Autodesk Inventor part; units mm, degrees
ref_plane "YZ Plane" through (0, 0, 0) normal (1, 0, 0) x (0, 1, 0)
ref_plane "XZ Plane" through (0, 0, 0) normal (0, 1, 0) x (-1, 0, 0)
ref_plane "XY Plane" through (0, 0, 0) normal (0, 0, 1) x (1, 0, 0)
sketch "Sketch1" plane through (0, 0, 0) normal (0, 0, 1) x (1, 0, 0)
  line L0 (0, 0) -> (95, 0)
  line L1 (95, 0) -> (95, 20)
  line L2 (95, 20) -> (0, 20)
  line L3 (0, 20) -> (0, 0)
  line L4 (8.5, 14.5) -> (14.5, 14.5)
  line L5 (18, 10.2244) -> (18, 9.7756)
  line L6 (14.5, 5.5) -> (8.5, 5.5)
  line L7 (5, 9.7756) -> (5, 10.2244)
  line L8 (11.5, 14.5) -> (8.5, 14.5)
  arc A0 (8.5, 14.5) -> (5, 10) centre (9.4986, 10.1122) ccw
  arc A1 (5, 10) -> (8.5, 5.5) centre (9.4986, 9.8878) ccw
  arc A2 (18, 10) -> (14.5, 14.5) centre (13.5014, 10.1122) ccw
  arc A3 (14.5, 5.5) -> (18, 10) centre (13.5014, 9.8878) ccw
  line L9 (86.5, 14.5) -> (80.5, 14.5)
  line L10 (77, 10.2244) -> (77, 9.7756)
  line L11 (80.5, 5.5) -> (86.5, 5.5)
  line L12 (90, 9.7756) -> (90, 10.2244)
  line L13 (83.5, 14.5) -> (86.5, 14.5)
  arc A4 (90, 10) -> (86.5, 14.5) centre (85.5014, 10.1122) ccw
  arc A5 (86.5, 5.5) -> (90, 10) centre (85.5014, 9.8878) ccw
  arc A6 (80.5, 14.5) -> (77, 10) centre (81.4986, 10.1122) ccw
  arc A7 (77, 10) -> (80.5, 5.5) centre (81.4986, 9.8878) ccw
  point P0 (47.5, 10)
  point P1 (11.5, 10)
  point P2 (83.5, 10)
  dimension "d0" = 95
  dimension "d1" = 20
extrude "Extrusion1" add sketch "Sketch1" along normal blind 2.5
sketch "Sketch2" plane through (0, 20, 0) normal (0, 1, 0) x (1, 0, 0)
  line L0 (0, 0) -> (95, 0)
  line L1 (47.5, 0) -> (21, 0)
  line L2 (47.5, 0) -> (74, 0) construction
  line L3 (47.5, 0) -> (74, 0)
  line L4 (47.5, 0) -> (74, 0) construction
  line L5 (74, 0) -> (74, -2.5)
  line L6 (0, -2.5) -> (95, -2.5)
  line L7 (21, 0) -> (21, -2.5)
  line L8 (21, -2.5) -> (74, -2.5)
extrude "Extrusion2" add sketch "Sketch2" along normal blind 12
sketch "Sketch3" plane through (0, 0, 2.5) normal (0, 0, 1) x (1, 0, 0)
  line L0 (74, 32) -> (21, 32)
  line L1 (0, 0) -> (95, 0)
  line L2 (21, 32) -> (23.5, 32)
  line L3 (23.5, 32) -> (23.5, 2.5)
  line L4 (23.5, 0) -> (21, 0)
  line L5 (21, 0) -> (21, 32)
  line L6 (74, 20) -> (74, 32)
  line L7 (74, 20) -> (74, 0)
  line L8 (74, 0) -> (71.5, 0)
  line L9 (71.5, 2.5) -> (71.5, 32)
  line L10 (71.5, 32) -> (74, 32)
  line L11 (74, 32) -> (74, 0)
  line L12 (23.5, 0) -> (71.5, 0)
  line L13 (71.5, 2.5) -> (23.5, 2.5)
extrude "Extrusion3" add sketch "Sketch3" along normal blind 30.5 contours L6 L7 L1 L5 L0 L3 L13 L9
sketch "Sketch4" plane through (23.5, 2.5, 2.5) normal (0, 1, 0) x (1, 0, 0)
  line L0 (48, -30.5) -> (0, -30.5)
  line L1 (48, 0) -> (48, -30.5)
  line L2 (0, -30.5) -> (48, -30.5)
  line L3 (48, -30.5) -> (48, -28)
  line L4 (48, -28) -> (0, -28)
  line L5 (0, -28) -> (0, -30.5)
  point P0 (-23.5, 2.5)
  dimension "d24" = 2.5
extrude "Extrusion4" add sketch "Sketch4" along normal up to surface (29.5 mm away)
sketch "Sketch5" plane through (23.5, 2.5, 2.5) normal (1, 0, 0) x (0, 0, -1)
  line L0 (0, 0) -> (-28, 0)
  line L1 (-14, 0) -> (-14, 29.5)
  line L2 (0, 29.5) -> (-28, 29.5)
  line L3 (-15, 14.75) -> (-15, 24.75)
  line L4 (-15, 14.75) -> (-15, 4.75)
  line L5 (-13, 14.75) -> (-13, 4.75)
  line L6 (-13, 14.75) -> (-13, 24.75)
  arc A0 (-13, 24.75) -> (-15, 24.75) centre (-14, 24.75) ccw
  arc A1 (-15, 4.75) -> (-13, 4.75) centre (-14, 4.75) ccw
  line L7 (-14, 14.75) -> (-14, 15.75)
  line L8 (-15, 14.75) -> (-13, 14.75)
  line L9 (-23, 14.75) -> (-23, 24.75)
  line L10 (-21, 14.75) -> (-21, 24.75)
  line L11 (-21, 14.75) -> (-21, 4.75)
  line L12 (-23, 14.75) -> (-23, 4.75)
  arc A2 (-23, 4.75) -> (-21, 4.75) centre (-22, 4.75) ccw
  arc A3 (-21, 24.75) -> (-23, 24.75) centre (-22, 24.75) ccw
  line L13 (-6, 14.75) -> (-6, 15.75)
  line L14 (-7, 14.75) -> (-7, 4.75)
  line L15 (-5, 14.75) -> (-5, 4.75)
  arc A4 (-7, 4.75) -> (-5, 4.75) centre (-6, 4.75) ccw
  line L16 (-7, 14.75) -> (-7, 24.75)
  line L17 (-5, 14.75) -> (-5, 24.75)
  arc A5 (-5, 24.75) -> (-7, 24.75) centre (-6, 24.75) ccw
  point P0 (2.5, -2.5)
  dimension "d38" = 8
  dimension "d45" = 8
extrude "Extrusion5" cut sketch "Sketch5" along normal through all both and the other way through all
sketch "Sketch8" plane through (71.5, 2.5, 30.5) normal (0, 0, -1) x (-1, 0, 0)
  line L0 (-2.5, 29.5) -> (50.5, 29.5)
  line L1 (48, 0) -> (0, 0)
  line L2 (24, 29.5) -> (53.5, 29.5) construction
  line L3 (23.9997, 15.0133) -> (24.9997, 15.0133) construction
  line L4 (22.9997, 15.0133) -> (22.9997, 25.0133)
  line L5 (22.9997, 15.0133) -> (22.9997, 5.0133)
  line L6 (24.9997, 15.0133) -> (24.9997, 5.0133)
  line L7 (24.9997, 15.0133) -> (24.9997, 25.0133)
  arc A0 (24.9997, 25.0133) -> (22.9997, 25.0133) centre (23.9997, 25.0393) ccw
  arc A1 (22.9997, 5.0133) -> (24.9997, 5.0133) centre (23.9997, 4.9873) ccw
  line L8 (30.9997, 15.0133) -> (30.9997, 25.0133)
  line L9 (30.9997, 15.0133) -> (30.9997, 5.0133)
  line L10 (32.9997, 15.0133) -> (32.9997, 5.0133)
  line L11 (32.9997, 15.0133) -> (32.9997, 25.0133)
  arc A2 (32.9997, 25.0133) -> (30.9997, 25.0133) centre (31.9997, 25.0393) ccw
  arc A3 (30.9997, 5.0133) -> (32.9997, 5.0133) centre (31.9997, 4.9873) ccw
  line L12 (38.9997, 15.0133) -> (38.9997, 25.0133)
  line L13 (38.9997, 15.0133) -> (38.9997, 5.0133)
  line L14 (40.9997, 15.0133) -> (40.9997, 5.0133)
  line L15 (40.9997, 15.0133) -> (40.9997, 25.0133)
  arc A4 (40.9997, 25.0133) -> (38.9997, 25.0133) centre (39.9997, 25.0393) ccw
  arc A5 (38.9997, 5.0133) -> (40.9997, 5.0133) centre (39.9997, 4.9873) ccw
  line L16 (14.9997, 15.0133) -> (14.9997, 25.0133)
  line L17 (16.9997, 15.0133) -> (16.9997, 25.0133)
  arc A6 (16.9997, 25.0133) -> (14.9997, 25.0133) centre (15.9997, 25.0393) ccw
  line L18 (14.9997, 15.0133) -> (14.9997, 5.0133)
  line L19 (16.9997, 15.0133) -> (16.9997, 5.0133)
  arc A7 (14.9997, 5.0133) -> (16.9997, 5.0133) centre (15.9997, 4.9873) ccw
  line L20 (6.9997, 15.0133) -> (6.9997, 25.0133)
  line L21 (8.9997, 15.0133) -> (8.9997, 25.0133)
  arc A8 (8.9997, 25.0133) -> (6.9997, 25.0133) centre (7.9997, 25.0393) ccw
  line L22 (6.9997, 15.0133) -> (6.9997, 5.0133)
  line L23 (8.9997, 15.0133) -> (8.9997, 5.0133)
  arc A9 (6.9997, 5.0133) -> (8.9997, 5.0133) centre (7.9997, 4.9873) ccw
  point P0 (71.5, -2.5)
  point P1 (31.9997, 15.0133)
  point P2 (39.9997, 15.0133)
  point P3 (15.9997, 15.0133)
  point P4 (22.9997, 25.0133)
  point P5 (24.9997, 25.0133)
  point P6 (7.9997, 15.0133)
  point P7 (14.9997, 25.0133)
  point P8 (15.9997, 25.0393)
  dimension "d64" = 8
  dimension "d71" = 8
extrude "Extrusion6" cut sketch "Sketch8" against normal up to surface (2.5 mm away)
fillet "Fillet1" radius 2 4 edges at (74, 16, 33) (21, 16, 33) (74, 26, 0) (21, 26, 0)
fillet "Fillet2" radius 2 5 edges at (73.4142, 0, 32.4142) (74, 0, 16.75) (21.5858, 0, 32.4142) (21, 0, 16.75) (47.5, 0, 33)
properties part number "SCDHolder3"
For this review, take the finished solid that the model builds, in its own axes (mm). A direction names the side the tool comes from. Round coordinates to 2 decimals unless told otherwise and drop trailing zeros. Order: outer loops, then holes, each group sorted by start corner. A loop starts at its lowest first (then second) coordinate and runs counter-clockwise, first axis right, second up. Notation, with made-up numbers: (42.25, 50) -> (53.25, 50) arc R17 cw to (53.25, 77) -> close; hole circle Ø10 at (78, 79.25). An arc over 180 degrees is marked (long way). Write item = value, one per line. Start each with the question number.
1) Tool access review of faces 1 (the face through (84, 14.5, 1)), 2 (the face through (63.523, 6.487, 31.732)), 3 (the face through (72.73, 28.25, 24.52)): name each direction out of +Z, -Z, +X, -X, +Y, -Y from which nothing blocks a thin tool from reaching the whole face with its end or side.
2) Take a section at C-C on z = 27.5. State the section outline as (x, y) points.
3) To check wall thickness, follow line 1 (Z direction, x = 23, y = 24); line 2 (Z direction, x = 25.5, y = 25); line 3 (X direction, y = 30.5, z = 25.5). State the ranges of each line that lie inside material, in increasing order. Write a range as from..to.
4) Take a section at B-B on x = 67.5. State the section outline as (y, z) points.
5) Take a section at D-D on y = 25. Count the separate pieces of the cut face and the enclosed holes in it, plus the area to 3 significant figures.
6) Insertion check: pin 1 (3 mm diameter, centred on x = 22.5, y = 15, fed in from +Z); pin 2 (3 mm diameter, centred on y = 15, z = 31.5, fed in from +X); pin 3 (0.8 mm diameter, centred on y = 14, z = 32, fed in from -X); pin 4 (1.2 mm diameter, centred on y = 14, z = 32.5, fed in from +X). Each pin has a flat end and moves straight along its axis. Give the tip position at first contact, or say it passes through.
7) Take a section at A-A on z = 8.5. State the section outline as (x, y) points.
8) The part is to be moulded in two halves that separate along Z. For faces 4 (the face through (47.84, 0.6, 32.43)), 5 (the face through (95, 10, 1)), 6 (the face through (47, 17, 2.5)), say which applies: +Z half, -Z half, draft (parallel to the pull), parting line (faces both ways), or undercut.
Verdict:
q1.face_1 = +Z, -Z
q1.face_2 = +Z
q1.face_3 = +X, -X
q2.outline = (21, 2) arc R2 ccw to (23, 0) -> (72, 0) arc R2 ccw to (74, 2) -> (74, 32) -> (71.5, 32) -> (71.5, 2.5) -> (23.5, 2.5) -> (23.5, 32) -> (21, 32) -> close
q3.line_1 = 0..7.5, 9.5..15.5, 17.5..23.5, 25.5..33
q3.line_2 = 0..2.5, 30.5..33
q3.line_3 = 21..23.5, 71.5..74
q4.outline = (0, 0) -> (32, 0) -> (32, 2.5) -> (2.5, 2.5) -> (2.5, 30.5) -> (32, 30.5) -> (32, 33) -> (2, 33) arc R2 ccw to (0, 31) -> close
q5.separate_pieces = 11
q5.enclosed_holes = 0
q5.area = 347 mm2
q6.pin_1 = 33
q6.pin_2 = 74
q6.pin_3 = 21.09
q6.pin_4 = 73.79
q7.outline = (21, 2) arc R2 ccw to (23, 0) -> (72, 0) arc R2 ccw to (74, 2) -> (74, 6.25) -> (71.5, 6.25) -> (71.5, 2.5) -> (23.5, 2.5) -> (23.5, 6.25) -> (21, 6.25) -> close; (21, 28.25) -> (23.5, 28.25) -> (23.5, 32) -> (21, 32) -> close; (71.5, 28.25) -> (74, 28.25) -> (74, 32) -> (71.5, 32) -> close
q8.face_4 = +Z half
q8.face_5 = draft
q8.face_6 = undercut
